```python
from build123d import *

# Parameters (mm, degrees)
F0_W     = 400
F0_H     = 352
F1_DEPTH = 19
F3_DEPTH = 19.001
F5_DEPTH = 19.0010001
F6_W     = 23.7784683704
F6_H     = 41.3538441062
F7_DEPTH = 19.0010001


with BuildPart() as f1:
    # F0 (on Top) → F1 (new body)
    with BuildSketch(Plane.XY):
        Rectangle(F0_W, F0_H)
    extrude(amount=F1_DEPTH)

    # F2 (on face) → F3 (cut, through all)
    with BuildSketch(Plane.XY.offset(19)):
        with BuildLine():
            add(Edge.make_bspline(
                [(-200, -31.5323062241), (-125.2770154333, -36.2490441097), (5.7780898117, -44.5216336427), (4.4484516613, -136.4751329034), (3.8769261446, -176)],
                knots=[0, 0, 0, 0, 0.5701646222, 1, 1, 1, 1], degree=3))
            Line((-200, -31.5323062241), (-200, -176))
            Line((-200, -176), (3.8769261446, -176))
        make_face()
        with BuildLine():
            Line((-200, 176), (-200, 33.0830775201))
            add(Edge.make_bspline(
                [(-200, 33.0830775201), (-124.0325945429, 34.1230566676), (10.5757099688, 35.9658184275), (3.2091678996, 133.5070419218), (0, 176)],
                knots=[0, 0, 0, 0, 0.5643589802, 1, 1, 1, 1], degree=3))
            Line((0, 176), (-200, 176))
        make_face()
        with BuildLine():
            ThreePointArc((200, -150.9415358305), (189.8823225958, -167.8969578857), (171.8769222498, -176))
            Line((171.8769222498, -176), (200, -176))
            Line((200, -176), (200, -150.9415358305))
        make_face()
    extrude(amount=-F3_DEPTH, mode=Mode.SUBTRACT)

    # F4 (on face) → F5 (cut, through all)
    with BuildSketch(Plane.XY.offset(19)):
        with BuildLine():
            ThreePointArc((177.4510932605, 176), (191.7387998266, 169.8211963235), (200, 156.6276848316))
            Line((200, 156.6276848316), (200, 176))
            Line((200, 176), (177.4510932605, 176))
        make_face()
    extrude(amount=-F5_DEPTH, mode=Mode.SUBTRACT)

    # F6 (on face) → F7 (cut, through all)
    with BuildSketch(Plane.XY.offset(19)):
        with Locations((-166.7076945305, 0)):
            Rectangle(F6_W, F6_H)
    extrude(amount=-F7_DEPTH, mode=Mode.SUBTRACT)


solid = f1.part
```
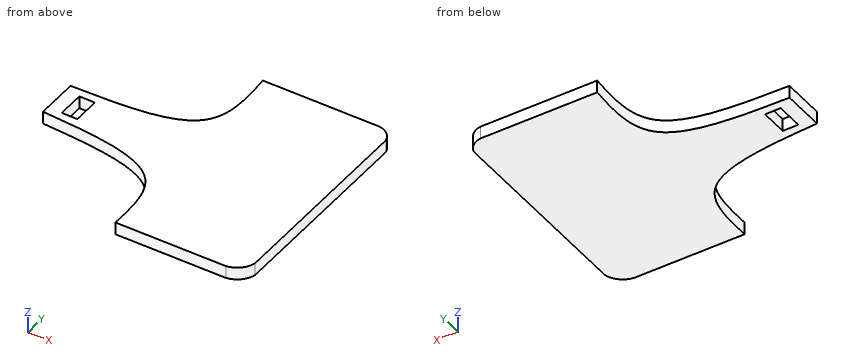
Design review of the part built by this model. Coordinates are the model's own, in mm. Coordinates: 2 decimals unless noted, no trailing zeros. Order: outer loops, then holes, each group sorted by start corner. A loop starts at its lowest first (then second) coordinate and runs counter-clockwise, first axis right, second up.
1) Clearance check with flat-ended pins moving along their axes: pin 1 (8 mm diameter, centred on x = -124.5, z = 16.5, fed in from -Y); pin 2 (1.5 mm diameter, centred on x = -106.5, z = 3, fed in from -Y); pin 3 (6 mm diameter, centred on x = -147, z = 8, fed in from +Y). State where each tip first meets the part, or that it passes through.
2) Take a section at A-A, the plane y = 10.5. Give the boundary of the cut face in (x, z), and give its area (3 significant figures).
3) Wall thickness on line 1 along X through (y, z) = (10, 6.75); line 2 along X through (y, z) = (128, 7.75); line 3 along Y through (x, z) = (-172.5, 18): over which ranges is each line inside the solid? List them lowest first.
Returned:
1. pin 1: stops at y = -37.99
1. pin 2: stops at y = -39.97
1. pin 3: stops at y = 34.33
2. outline: (-200, 0) - (-178.6, 0) - (-178.6, 19) - (-200, 19) - close; (-154.82, 0) - (200, 0) - (200, 19) - (-154.82, 19) - close
2. area: 7,150 mm2
3. line 1: x = -200 to -178.6, -154.82 to 200
3. line 2: x = 2.17 to 200
3. line 3: y = -33.32 to -20.68, 20.68 to 33.51
